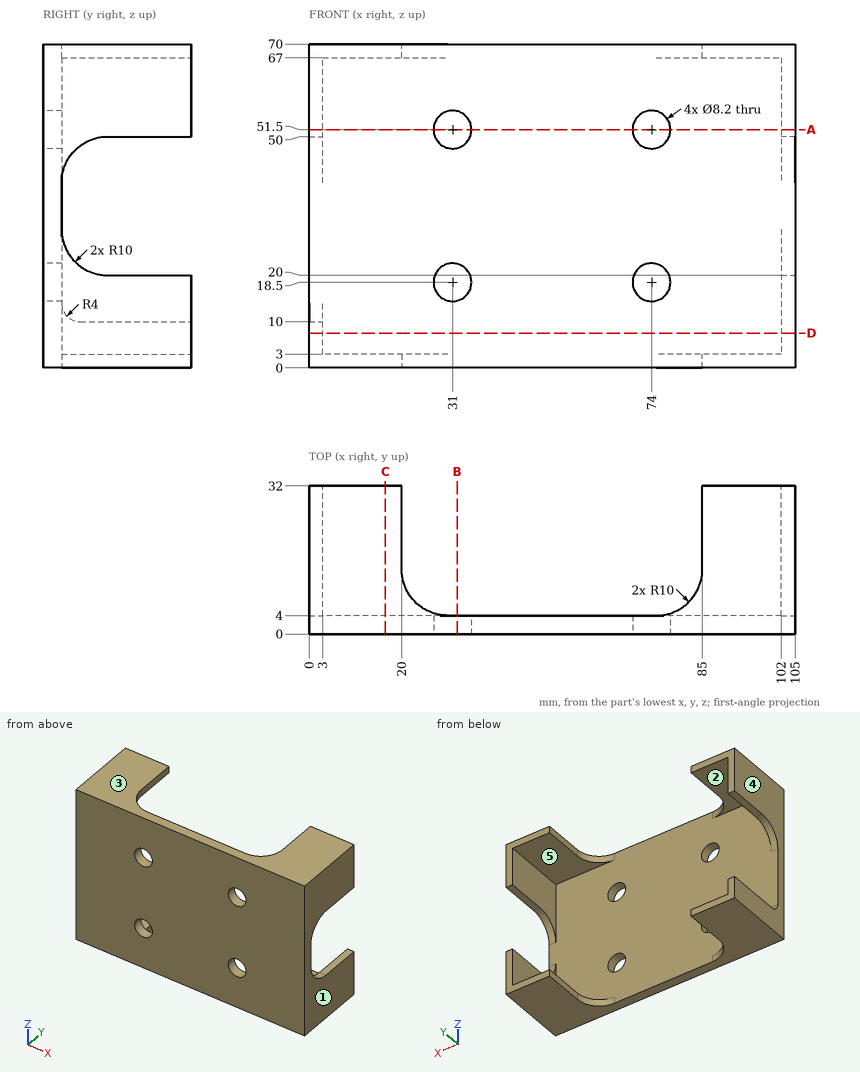
Part print with two shaded views. Sizes in mm from the minimum x, y, z corner. A direction names the side the tool comes from. Round coordinates to 2 decimals unless told otherwise and drop trailing zeros. Loops run counter-clockwise (first coordinate to the right, second up) from the corner with the lowest first, then second, coordinate; pieces in that order, holes last. Notation, with made-up numbers: M 87,43 L 106,43 A21 ccw 106,56 Z; hole C 32,-4 d10. An arc over 180 degrees is marked long. Put each result on its own line as item: value. Start each with the question number.
Item 1: Cut at D-D (z = 7.5). List the corners of the cut face in (x, y).
Item 2: Drop a flat-ended pin along its axis: P1, Ø6, axis at x = 92.5, z = 19.5, coming from the +Y side. Give the stop position or say it passes through.
Item 3: Cut at B-B (x = 32). List the corners of the cut face in (y, z), then the cut area to 3 significant figures.
Item 4: 3-axis set-ups, long thin cutter, end or side, ignore diameter. For the marked faces 4 and 5: which of +Z, -Z, +X, -X, +Y, -Y reach the whole face in a straight line?
Item 5: Cut at A-A (z = 51.5). List the corners of the cut face in (x, y).
Item 6: Cut at C-C (x = 16.5). List the corners of the cut face in (y, z), then the cut area to 3 significant figures.
Item 7: Mould opens along X. For the marked faces 1, 2 and 3 say: released by +X, released by -X, zero draft, split by the parting line, or undercut.
Item 8: Drill centre lines: line 1 along Z through (x, y) = (74, 1.9); line 2 along Z through (x, y) = (90.5, 21); line 3 along X through (y, z) = (19.5, 53). Where is each one in solid material? Low to high.
Answer block:
1. outline: M 0,0 L 105,0 L 105,32 L 102,32 L 102,4 L 3,4 L 3,32 L 0,32 Z
2. P1: y = 4
3. outline: M 0,0 L 4,0 L 4,14.52 L 0,14.52 Z; M 0,22.48 L 4,22.48 L 4,47.52 L 0,47.52 Z; M 0,55.48 L 4,55.48 L 4,70 L 0,70 Z
3. area: 216 mm2
4. face 4: +Z, -Z, -X, +Y, -Y
4. face 5: +Y
5. outline: M 0,0 L 26.9,0 L 26.9,4 L 3,4 L 3,32 L 0,32 Z; M 35.1,0 L 69.9,0 L 69.9,4 L 35.1,4 Z; M 78.1,0 L 105,0 L 105,32 L 102,32 L 102,4 L 78.1,4 Z
6. outline: M 0,0 L 32,0 L 32,3 L 4,3 L 4,67 L 32,67 L 32,70 L 0,70 Z
6. area: 448 mm2
7. face 1: released by +X
7. face 2: undercut
7. face 3: zero draft
8. line 1: 0 to 14.4, 22.6 to 47.4, 55.6 to 70
8. line 2: 0 to 3, 67 to 70
8. line 3: 0 to 3, 102 to 105
